Part model, mm, in its own coordinate system. A direction names the side the tool comes from. Round coordinates to 2 decimals unless told otherwise and drop trailing zeros. Write each loop counter-clockwise with the first axis right and the second up, starting at its lowest first coordinate (ties: lowest second). Pieces come first, ordered by that corner, then holes. Notation, with made-up numbers: (-30, -9) -> (12, -9) arc R21 ccw to (12, 8) -> close; hole circle Ø8 at (60.5, 61). An arc over 180 degrees is marked (long way). Return JSON: item names as keys, results as strings. Group by question number.
(1) Drop flat-ended pins along their axis: pin 1 Ø11 at (x, y) = (37.5, 8.5) entering from +Z; pin 2 Ø13 at (y, z) = (-5.5, -2.5) entering from +X. Give the stop position or say it passes through.
(2) Mould opens along Z. For faces 1 (the cylindrical face through (8.57, 0.25, -20.75)), 2 (the flat face through (8, 0, 1)), 3 (the flat face through (53, 0, -22.25)) say: +Z half, -Z half, draft (parallel to the pull), parting line (faces both ways), or undercut.
(3) Saw through at C-C (x = 54.5). List the corners of the cut face in (y, z), plus the area to 3 significant figures.
(4) Tool access for faces 4 (the cylindrical face through (88, 0.25, -20.78)), 5 (the flat face through (48, -21.5, 0)): list every direction of +Z, -Z, +X, -X, +Y, -Y with a clear straight run to the whole face (end or side of a thin tool).
(5) Saw through at B-B (y = 11). List the corners of the cut face in (x, z), plus the area to 3 significant figures.
(6) Drill centre lines: L1, parallel to Y at x = 74.5, z = 9.5; L2, parallel to X at y = 14, z = 18.5; L3, parallel to Z at x = 35, y = -16. Where is each one in solid material? Low to high. Write a range as from..to.
(7) Saw through at A-A (z = 15). List the corners of the cut face in (x, y).
(8) Saw through at D-D (y = -5). List the corners of the cut face in (x, z), plus the area to 3 significant figures.
from build123d import *

# Parameters (mm, degrees)
SKETCH_1_W                  = 86
SKETCH_1_H                  = 43
EXTRUDE_1_DEPTH             = 39.5
EXTRUDE_2_DEPTH             = 5
SKETCH_3_W                  = 80.6
SKETCH_3_H                  = 40.2
CUT_EXTRUDE_1_DEPTH         = 43.6
HOLE_WIZARD_8_3_8_3_1_D     = 8.3
HOLE_WIZARD_8_3_8_3_1_DEPTH = 3.2
FILLET_1_R                  = 3
EXTRUDE_START               = -4
SKETCH_6_R                  = 4.15
EXTRUDE_3_DEPTH             = 4
FILLET_2_R                  = 2


with BuildPart() as part:
    # Эскиз1 → Бобышка-Вытянуть1 (new body)
    with BuildSketch(Plane.XY.offset(22.25)):
        with Locations((47, 0)):
            Rectangle(SKETCH_1_W, SKETCH_1_H)
    extrude(amount=-EXTRUDE_1_DEPTH)

    # Эскиз2 → Бобышка-Вытянуть2 (add)
    with BuildSketch(Plane(origin=(0, 0, -17.25), x_dir=(-1, 0, 0), z_dir=(0, 0, -1))):
        with BuildLine():
            Line((-90, -21.5), (-90, -16.5))
            ThreePointArc((-90, -16.5), (-104, 0), (-90, 16.5))
            Line((-90, 16.5), (-90, 21.5))
            Line((-90, 21.5), (-4, 21.5))
            Line((-4, 21.5), (-4, -21.5))
            Line((-4, -21.5), (-90, -21.5))
        make_face()
        with BuildLine():
            Line((-90, -12.428366172), (-90, 12.428366172))
            ThreePointArc((-90, 12.428366172), (-100, 0), (-90, -12.428366172))
        make_face(mode=Mode.SUBTRACT)
    extrude(amount=EXTRUDE_2_DEPTH)

    # Эскиз3 → Вырез-Вытянуть1 (cut)
    with BuildSketch(Plane.XY.offset(22.25)):
        with Locations((48.3, 0)):
            Rectangle(SKETCH_3_W, SKETCH_3_H)
    extrude(amount=-CUT_EXTRUDE_1_DEPTH, mode=Mode.SUBTRACT)

    # Диаметр отверстия Ø8.3 (8.3)1
    with Locations(Plane.ZY.offset(-4)):
        with Locations((0, 0)):
            Hole(HOLE_WIZARD_8_3_8_3_1_D / 2, depth=HOLE_WIZARD_8_3_8_3_1_DEPTH)

    # Скругление1
    fillet_1_edges = [part.edges().sort_by_distance(p)[0] for p in [
        (4, -21.5, 0),
        (4, 21.5, 0),
    ]]
    fillet(fillet_1_edges, radius=FILLET_1_R)

    # Эскиз6 → Бобышка-Вытянуть3 (add)
    with BuildSketch(Plane.ZY.offset(-4).offset(EXTRUDE_START)):
        Circle(SKETCH_6_R)
    extrude(amount=EXTRUDE_3_DEPTH)

    # Скругление2
    fillet_2_edges = [part.edges().sort_by_distance(p)[0] for p in [
        (48.3, -20.1, -21.35),
        (88.6, -20.1, 0.45),
        (8, 0, -21.35),
        (8, -20.1, 0.45),
        (48.3, 20.1, -21.35),
        (8, 20.1, 0.45),
        (88.6, 0, -21.35),
        (88.6, 20.1, 0.45),
    ]]
    fillet(fillet_2_edges, radius=FILLET_2_R)


solid = part.part
Computed values:
{
 "1": {"pin 1": "z = -21.35", "pin 2": "x = 90"},
 "2": {"face 1": "+Z half", "face 2": "draft", "face 3": "-Z half"},
 "3": {"outline": "(-21.5, -22.25) -> (21.5, -22.25) -> (21.5, 22.25) -> (20.1, 22.25) -> (20.1, -19.35) arc R2 cw to (18.1, -21.35) -> (-18.1, -21.35) arc R2 cw to (-20.1, -19.35) -> (-20.1, 22.25) -> (-21.5, 22.25) -> close", "area": "162 mm2"},
 "4": {"face 4": "+Z", "face 5": "+Z, -Z, +X, -X, -Y"},
 "5": {"outline": "(4, -22.25) -> (90, -22.25) -> (90, 22.25) -> (88.6, 22.25) -> (88.6, -19.35) arc R2 cw to (86.6, -21.35) -> (10, -21.35) arc R2 cw to (8, -19.35) -> (8, 22.25) -> (4, 22.25) -> close; (93.67, -22.25) -> (99.87, -22.25) -> (99.87, -17.25) -> (93.67, -17.25) -> close", "area": "346 mm2"},
 "6": {"L1": "-21.5..-20.1, 20.1..21.5", "L2": "4..8, 88.6..90", "L3": "-22.25..-21.35"},
 "7": {"outline": "(4, -18.5) arc R3 ccw to (7, -21.5) -> (90, -21.5) -> (90, 21.5) -> (7, 21.5) arc R3 ccw to (4, 18.5) -> close; hole (8, -18.1) arc R2 ccw to (10, -20.1) -> (86.6, -20.1) arc R2 ccw to (88.6, -18.1) -> (88.6, 18.1) arc R2 ccw to (86.6, 20.1) -> (10, 20.1) arc R2 ccw to (8, 18.1) -> close"},
 "8": {"outline": "(4, -22.25) -> (90, -22.25) -> (90, 22.25) -> (88.6, 22.25) -> (88.6, -19.35) arc R2 cw to (86.6, -21.35) -> (10, -21.35) arc R2 cw to (8, -19.35) -> (8, 22.25) -> (4, 22.25) -> close; (98.98, -22.25) -> (103.24, -22.25) -> (103.24, -17.25) -> (98.98, -17.25) -> close", "area": "336 mm2"}
}
